Build history of the part. All positions in model axes, mm. Round coordinates to 2 decimals unless told otherwise and drop trailing zeros. Order: outer loops, then holes, each group sorted by start corner. A loop starts at its lowest first (then second) coordinate and runs counter-clockwise, first axis right, second up. Notation, with made-up numbers: (26.5, 15.5) - (35.5, 15.5) arc R15 cw to (35.5, 35.5) - close; hole circle Ø8 at (69.25, 8.25). An arc over 180 degrees is marked (long way). Write each question's results on one line, items separated by ' | '. Start each with the question number.
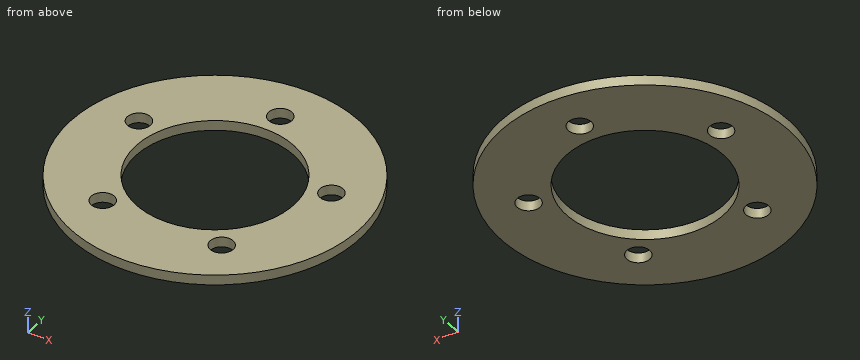
```python
from build123d import *

# Parameters (mm, degrees)
SKETCH1_R           = 22.86
SKETCH1_R_2         = 12.5
SKETCH1_R_3         = 1.8288
BOSS_EXTRUDE1_DEPTH = 1.5875


with BuildPart() as part:
    # Sketch1 → Boss-Extrude1 (new body)
    with BuildSketch(Plane(origin=(0, 0, -12.7), x_dir=(-1, 0, 0), z_dir=(0, 0, -1))):
        Circle(SKETCH1_R)
        Circle(SKETCH1_R_2, mode=Mode.SUBTRACT)
        with Locations((15.216904261, 4.94427191)):
            Circle(SKETCH1_R_3, mode=Mode.SUBTRACT)
        with Locations((9.404564037, -12.94427191)):
            Circle(SKETCH1_R_3, mode=Mode.SUBTRACT)
        with Locations((-9.404564037, -12.94427191)):
            Circle(SKETCH1_R_3, mode=Mode.SUBTRACT)
        with Locations((-15.216904261, 4.94427191)):
            Circle(SKETCH1_R_3, mode=Mode.SUBTRACT)
        with Locations((0, 16)):
            Circle(SKETCH1_R_3, mode=Mode.SUBTRACT)
    extrude(amount=BOSS_EXTRUDE1_DEPTH)


solid = part.part
```
1. Cut at A-A (x = 0). List the corners of the cut face in (y, z).
2. Cut at D-D (x = 14.5). List the corners of the cut face in (y, z), plus the area to 3 significant figures.
3. Cut at C-C (z = -14). List the corners of the cut face in (x, y).
4. Cut at B-B (y = 0). List the corners of the cut face in (x, z), plus the area to 3 significant figures.
5. Wall check: line 1 (Y direction, x = 0, z = -13.15); line 2 (X direction, y = 5, z = -13.75); line 3 (X direction, y = 2.5, z = -13.15). Give the ranges that are in metal, low to high. Write a range as from..to.
A:
1) outline: (-22.86, -14.29) - (-12.5, -14.29) - (-12.5, -12.7) - (-22.86, -12.7) - close; (12.5, -14.29) - (14.17, -14.29) - (14.17, -12.7) - (12.5, -12.7) - close; (17.83, -14.29) - (22.86, -14.29) - (22.86, -12.7) - (17.83, -12.7) - close
2) outline: (-17.67, -14.29) - (3.26, -14.29) - (3.26, -12.7) - (-17.67, -12.7) - close; (6.63, -14.29) - (17.67, -14.29) - (17.67, -12.7) - (6.63, -12.7) - close | area: 50.8 mm^2
3) outline: circle Ø45.72 at (0, 0); hole circle Ø3.66 at (-15.22, 4.94); hole circle Ø25 at (0, 0); hole circle Ø3.66 at (-9.4, -12.94); hole circle Ø3.66 at (0, 16); hole circle Ø3.66 at (9.4, -12.94); hole circle Ø3.66 at (15.22, 4.94)
4) outline: (-22.86, -14.29) - (-12.5, -14.29) - (-12.5, -12.7) - (-22.86, -12.7) - close; (12.5, -14.29) - (22.86, -14.29) - (22.86, -12.7) - (12.5, -12.7) - close | area: 32.9 mm^2
5) line 1: y = -22.86..-12.5, 12.5..14.17, 17.83..22.86 | line 2: x = -22.31..-17.04, -13.39..-11.46, 11.46..13.39, 17.04..22.31 | line 3: x = -22.72..-12.25, 12.25..22.72
